Source: three-view drawing plus pictorial views. Frame: mm from the lowest corner of the part. Give positions to 0.01 mm unless a question says otherwise; leave off trailing zeros. One line per item, written item: value.
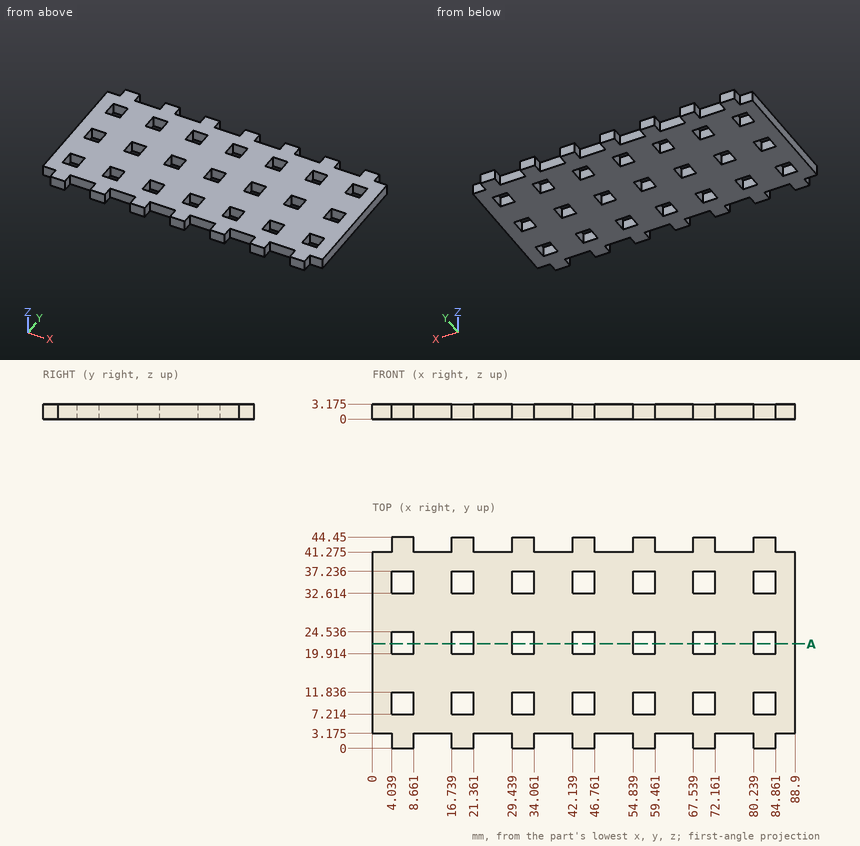
Item 1: Pin query (flat end, axial travel): P1, Ø1, axis at y = 35, z = 1.5, coming from the -X side. Return the tip coordinate at first contact, or that it passes through.
Verdict:
P1: stops at x = 0
Item 2: Section A-A, the plane y = 22. Count the separate pieces of the cut face and the enclosed holes in it.
Verdict:
separate pieces: 8
enclosed holes: 0
Item 3: Material intervals for L1, parallel to Y at x = 44, z = 2.15; L2, parallel to Y at x = 60.5, z = 2.35 (1 decimal), sorted ascending.
Verdict:
L1: y = 0 to 7.21, 11.84 to 19.91, 24.54 to 32.61, 37.24 to 44.45
L2: y = 3.2 to 41.3
